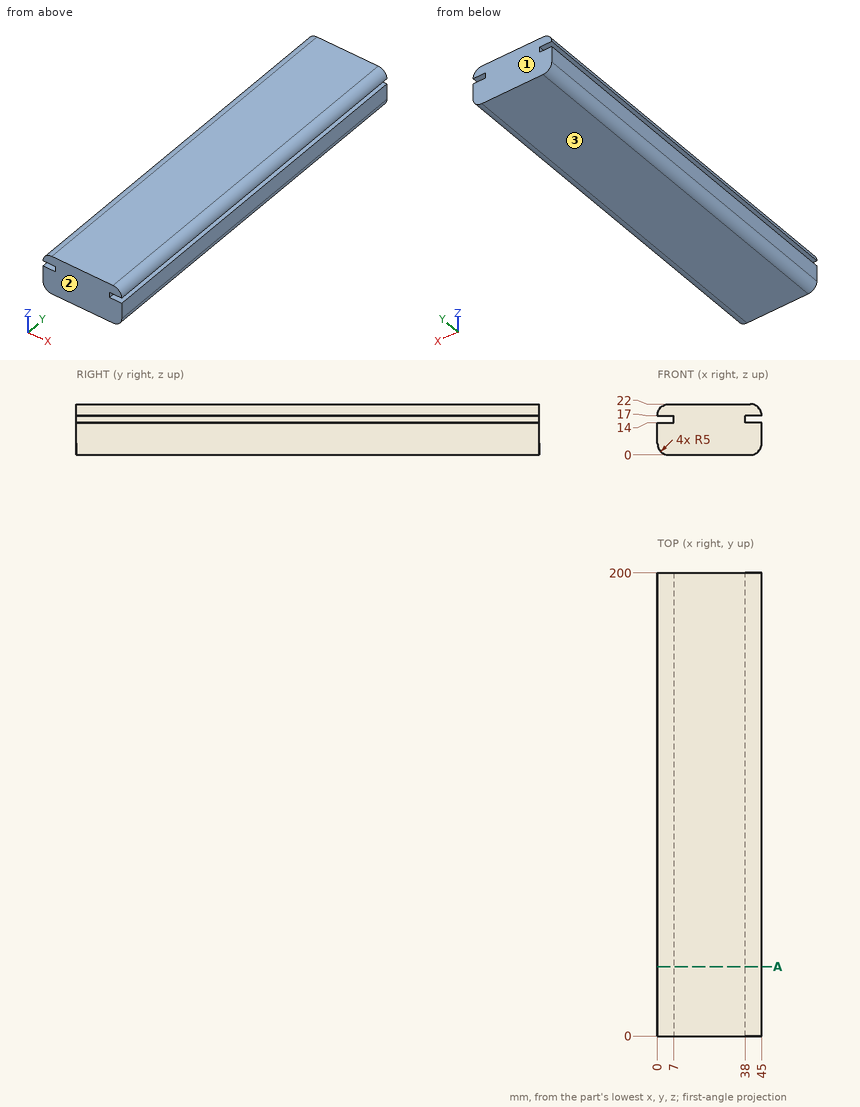
Design review of the part shown in the three views and the two pictorial views. Dimensions are in mm from the part's minimum x, y and z. Round coordinates to 2 decimals unless told otherwise and drop trailing zeros. Write each loop counter-clockwise with the first axis right and the second up, starting at its lowest first coordinate (ties: lowest second). Pieces come first, ordered by that corner, then holes.
Item 1: For pin 1 Ø2 at (x, y) = (3.5, 108) entering from +Z; pin 2 Ø2 at (x, y) = (42, 93.5) entering from +Z, all flat-tipped, find the tip position at first contact; note any pin that passes through.
Item 2: Consider section A-A on y = 30. Give the boundary of the cut face in (x, z), and give its area (3 significant figures).
Item 3: Draft analysis for pull direction Y (two halves, no side actions). For the marked faces 1, 2 and 3, state which applies: released by +Y, released by -Y, zero draft, split by the parting line, or undercut.
Item 4: Wall thickness on L1, parallel to Z at x = 40.5, y = 190; L2, parallel to Z at x = 43, y = 179.5; L3, parallel to X at y = 52.5, z = 15.5: over which ranges is each line inside the solid? List them lowest first.
Check values:
1. pin 1: stops at z = 21.97
1. pin 2: stops at z = 21.9
2. outline: (0, 5) arc R5 ccw to (5, 0) - (40, 0) arc R5 ccw to (45, 5) - (45, 14) - (38, 14) - (38, 17) - (45, 17) arc R5 ccw to (40, 22) - (5, 22) arc R5 ccw to (0, 17) - (7, 17) - (7, 14) - (0, 14) - close
2. area: 927 mm2
3. face 1: released by +Y
3. face 2: released by -Y
3. face 3: zero draft
4. L1: z = 0.03 to 14, 17 to 21.97
4. L2: z = 1 to 14, 17 to 21
4. L3: x = 7 to 38
